Check sheet for the modelled part. Datum: model origin and axes. Units: mm. A direction names the side the tool comes from. Coordinates: 2 decimals unless noted, no trailing zeros. Write each loop counter-clockwise with the first axis right and the second up, starting at its lowest first coordinate (ties: lowest second). Pieces come first, ordered by that corner, then holes. Notation, with made-up numbers: M 68,40.25 L 81,40.25 A30 cw 81,77.25 Z; hole C -39.5,79.25 d10. An arc over 180 degrees is marked long. Answer as CSV lines item,"result". Start each with the question number.
1) Section check B-B (y = 23). Record the cut outline in (x, z), and give its area (3 significant figures).
2) Section check C-C (x = 30). Record the cut outline in (y, z), and give its area (3 significant figures).
3) Go/stop test with flat-tipped pins: pin 1 Ø7 at (y, z) = (144, 1) entering from +X; pin 2 Ø2 at (y, z) = (104, -7) entering from +X; pin 3 Ø5 at (x, y) = (44, 112) entering from -Z; pin 4 Ø6 at (x, y) = (3.5, 48) entering from -Z. Record where each tip stops, or that it passes through.
4) Material ranges on L1, parallel to Y at x = 49.5, z = 0; L2, parallel to Y at x = 50, z = 0; L3, parallel to Z at x = -1, y = 49, recorded low to high. Write a range as [from, to].
5) Section check D-D (y = 4). State how many separate pieces and enclosed holes the cut face has, and give its area (3 significant figures).
6) Access from +Z, -Z, +X, -X, +Y, -Y to the whole of each face (thin tool, end or side, straight path). Record for faces 4 (the cylindrical face through (46.156, 73.457, -16.45)), 5 (the flat face through (49.7, 2.6, -1.4)), 6 (the flat face through (37.17, 2.6, -33.02)).
7) Section check A-A (z = 0). Record the cut outline in (x, y), and give its area (3 significant figures).
8) Draft check along Y on faces 1 (the flat face through (47.86, 73.46, 9.62)), 2 (the flat face through (38, 0, -33)), 3 (the cylindrical face through (38.92, 4.077, -30.375)). Enter one of: +Y half, -Y half, draft (parallel to the pull), parting line (faces both ways), or undercut.
from build123d import *

# Parameters (mm, degrees)
EXTRUDE_2_DEPTH          = 149
SKETCH_15_R              = 3.25
CUT_EXTRUDE_5_DEPTH      = 1.3
SKETCH_16_R              = 1.75
CUT_EXTRUDE_6_DEPTH      = 167.38914097
PATTERN_CIRCULAR_3_COUNT = 5
PATTERN_CIRCULAR_3_ANGLE = 80
SKETCH_17_R              = 3.25
CUT_EXTRUDE_7_DEPTH      = 1.3
SKETCH_18_R              = 1.75
CUT_EXTRUDE_8_DEPTH      = 167.389141002
PATTERN_CIRCULAR_5_COUNT = 5
PATTERN_CIRCULAR_5_ANGLE = 80


with BuildPart() as part:
    # Эскиз2 → Бобышка-Вытянуть2 (new body)
    with BuildSketch(Plane(origin=(0, 0, 0), x_dir=(1, 0, 0), z_dir=(0, 1, 0))):
        with BuildLine():
            Line((47.135590279, -12.793597189), (48.266574667, -13.051351269))
            ThreePointArc((48.266574667, -13.051351269), (48.75, -11.110243022), (49.155394108, -9.151351269))
            Line((49.155394108, -9.151351269), (50.131159715, -9.373730613))
            ThreePointArc((50.131159715, -9.373730613), (39.236846594, 32.580206711), (0, 51))
            Line((0, 51), (0, 50))
            ThreePointArc((0, 50), (-2, 49.959983987), (-3.996798719, 49.84))
            Line((-3.996798719, 49.84), (-3.996798719, 48.836723887))
            ThreePointArc((-3.996798719, 48.836723887), (12.196177114, 47.457910445), (27.047555214, 40.858655839))
            Line((27.047555214, 40.858655839), (33.952444786, 35.330319742))
            ThreePointArc((33.952444786, 35.330319742), (46.263287314, 16.146462365), (48.562738521, -6.531495034))
            Line((48.562738521, -6.531495034), (47.135590279, -12.793597189))
        make_face()
    extrude(amount=EXTRUDE_2_DEPTH)

    # Эскиз15 → Вырез-Вытянуть5 (cut)
    with BuildSketch(Plane(origin=(51, 0, 0), x_dir=(0, 0, -1), z_dir=(1, 0, 0))):
        with Locations((0, 4)):
            Circle(SKETCH_15_R)
    cut_extrude_5 = extrude(amount=-CUT_EXTRUDE_5_DEPTH, mode=Mode.SUBTRACT)

    # Эскиз16 → Вырез-Вытянуть6 (cut, through all)
    with BuildSketch(Plane(origin=(49.7, 0, 0), x_dir=(0, 0, -1), z_dir=(1, 0, 0))):
        with Locations((0, 4)):
            Circle(SKETCH_16_R)
    cut_extrude_6 = extrude(amount=-CUT_EXTRUDE_6_DEPTH, mode=Mode.SUBTRACT)

    # Круговой массив3: Вырез-Вытянуть5, Вырез-Вытянуть6 ×5 about axis, 2 skipped
    pattern_circular_3_axis = Axis((0, 0, 0), (0, 1, 0))
    add([cut_extrude_5.rotate(pattern_circular_3_axis, i * PATTERN_CIRCULAR_3_ANGLE / (PATTERN_CIRCULAR_3_COUNT - 1)) for i in range(1, PATTERN_CIRCULAR_3_COUNT) if i not in (1, 3)], mode=Mode.SUBTRACT)
    add([cut_extrude_6.rotate(pattern_circular_3_axis, i * PATTERN_CIRCULAR_3_ANGLE / (PATTERN_CIRCULAR_3_COUNT - 1)) for i in range(1, PATTERN_CIRCULAR_3_COUNT) if i not in (1, 3)], mode=Mode.SUBTRACT)

    # Эскиз17 → Вырез-Вытянуть7 (cut)
    with BuildSketch(Plane(origin=(51, 0, 0), x_dir=(0, 0, -1), z_dir=(1, 0, 0))):
        with Locations((0, 145)):
            Circle(SKETCH_17_R)
    cut_extrude_7 = extrude(amount=-CUT_EXTRUDE_7_DEPTH, mode=Mode.SUBTRACT)

    # Эскиз18 → Вырез-Вытянуть8 (cut, through all)
    with BuildSketch(Plane(origin=(49.7, 0, 0), x_dir=(0, 0, -1), z_dir=(1, 0, 0))):
        with Locations((0, 145)):
            Circle(SKETCH_18_R)
    cut_extrude_8 = extrude(amount=-CUT_EXTRUDE_8_DEPTH, mode=Mode.SUBTRACT)

    # Круговой массив5: Вырез-Вытянуть7, Вырез-Вытянуть8 ×5 about axis, 2 skipped
    pattern_circular_5_axis = Axis((0, 149, 0), (0, 1, 0))
    add([cut_extrude_7.rotate(pattern_circular_5_axis, i * PATTERN_CIRCULAR_5_ANGLE / (PATTERN_CIRCULAR_5_COUNT - 1)) for i in range(1, PATTERN_CIRCULAR_5_COUNT) if i not in (1, 3)], mode=Mode.SUBTRACT)
    add([cut_extrude_8.rotate(pattern_circular_5_axis, i * PATTERN_CIRCULAR_5_ANGLE / (PATTERN_CIRCULAR_5_COUNT - 1)) for i in range(1, PATTERN_CIRCULAR_5_COUNT) if i not in (1, 3)], mode=Mode.SUBTRACT)


solid = part.part
Results found:
1,outline,"M -4,-49.84 A50 ccw 0,-50 L 0,-51 A51 ccw 50.13,9.37 L 49.16,9.15 A50 ccw 48.27,13.05 L 47.14,12.79 L 48.56,6.53 A49 cw 33.95,-35.33 L 27.05,-40.86 A49 cw -4,-48.84 Z"
1,area,"186 mm2"
2,outline,"M 0,-41.24 L 149,-41.24 L 149,-38.49 L 0,-38.49 Z"
2,area,"410 mm2"
3,pin 1,"stops at x = 51"
3,pin 2,"stops at x = 50.65"
3,pin 3,"stops at z = -29.64"
3,pin 4,"stops at z = -51"
4,L1,"y = [0, 2.25], [5.75, 143.25], [146.75, 149]"
4,L2,"y = [0, 0.75], [7.25, 141.75], [148.25, 149]"
4,L3,"z = [-49.99, -48.99]"
5,separate pieces,"4"
5,enclosed holes,"0"
5,area,"153 mm2"
6,face 4,"-X, +Y, -Y"
6,face 5,"+X"
6,face 6,"none"
7,outline,"M 49,0 L 51,0 L 51,0.75 L 49.7,0.75 L 49.7,2.25 L 49,2.25 Z; M 49,5.75 L 49.7,5.75 L 49.7,7.25 L 51,7.25 L 51,141.75 L 49.7,141.75 L 49.7,143.25 L 49,143.25 Z; M 49,146.75 L 49.7,146.75 L 49.7,148.25 L 51,148.25 L 51,149 L 49,149 Z"
7,area,"276 mm2"
8,face 1,"draft"
8,face 2,"-Y half"
8,face 3,"undercut"
